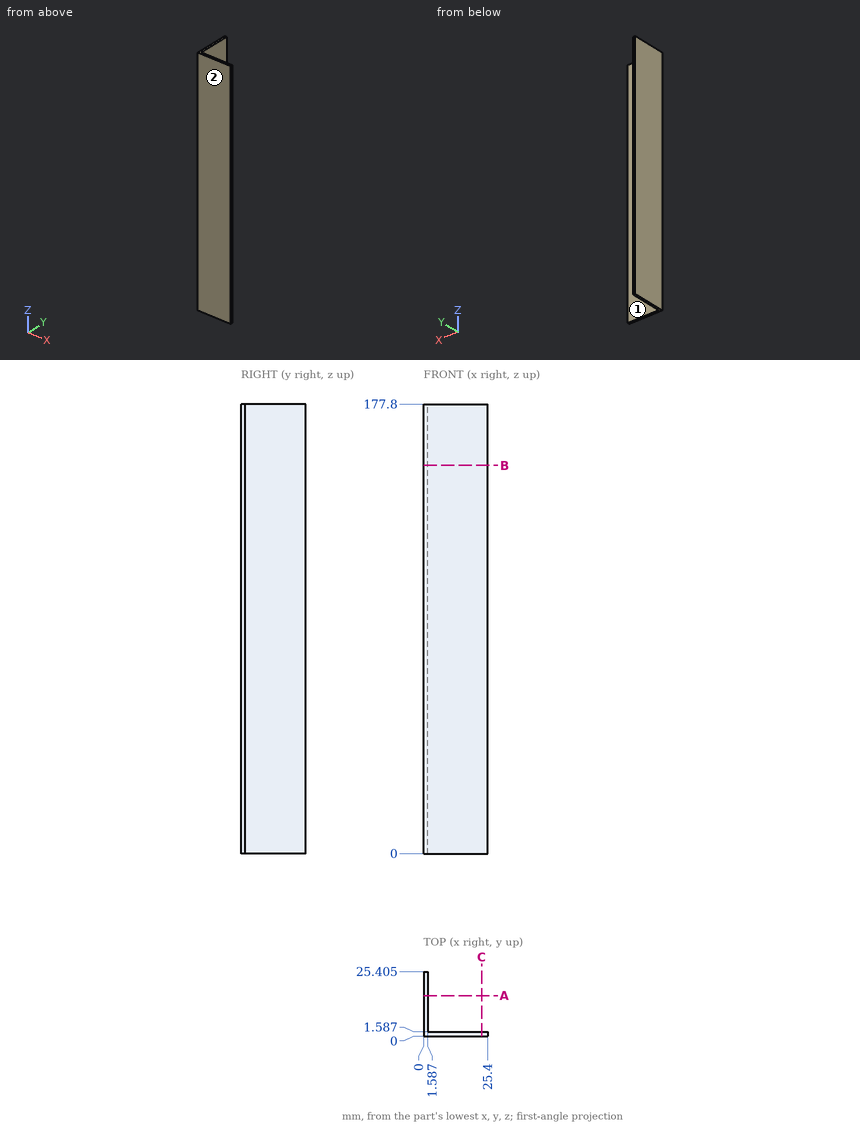
Design review of the part shown in the three views and the two pictorial views. Dimensions are in mm from the part's minimum x, y and z. A direction names the side the tool comes from. Round coordinates to 2 decimals unless told otherwise and drop trailing zeros. Write each loop counter-clockwise with the first axis right and the second up, starting at its lowest first coordinate (ties: lowest second). Pieces come first, ordered by that corner, then holes. Notation, with made-up numbers: (55, 83.25) - (66, 83.25) arc R22 ccw to (66, 100.25) - close; hole circle Ø6 at (82.25, 14). An arc over 180 degrees is marked (long way). Write item = value, one per line. Start each with the question number.
1. Wall thickness on L1, parallel to Y at x = 8.25, z = 41: over which ranges is the line inside the solid? List them lowest first.
2. Consider section A-A on y = 16. State the section outline as (x, z) points.
3. For the marked faces 1 and 2, list the 3-axis set-ups (+Z, -Z, +X, -X, +Y, -Y) from which the entire face can be reached by the end or side of a thin tool; tool diameter is ignored.
4. For pin 1 Ø6 at (x, z) = (17, 31.5) entering from +Y; pin 2 Ø5 at (y, z) = (11, 113.5) entering from +X, all flat-tipped, find the tip position at first contact; note any pin that passes through.
5. Consider section B-B on z = 153.5. State the section outline as (x, y) points (1 decimal).
Evaluation:
q1.L1 = 0 to 1.59
q2.outline = (0, 0) - (1.59, 0) - (1.59, 177.8) - (0, 177.8) - close
q3.face_1 = +Z, -Z, +X, +Y
q3.face_2 = +Z, -Z, +X, -X, -Y
q4.pin_1 = 1.59
q4.pin_2 = 1.59
q5.outline = (0, 0) - (25.4, 0) - (25.4, 1.6) - (1.6, 1.6) - (1.6, 25.4) - (0, 25.4) - close
